Verification items for the finished model (mm, model axes). Face numbers are marked on the shaded views. A direction names the side the tool comes from. Round coordinates to 2 decimals unless told otherwise and drop trailing zeros. Order: outer loops, then holes, each group sorted by start corner. A loop starts at its lowest first (then second) coordinate and runs counter-clockwise, first axis right, second up. Notation, with made-up numbers: M 18,20 L 34,20 A17 cw 34,25 Z; hole C 23,39.25 d6. An arc over 180 degrees is marked long. Return JSON: item names as keys, results as strings. Group by question number.
from build123d import *

# Parameters (mm, degrees)
SKETCH1_R           = 2.5
BOSS_EXTRUDE1_DEPTH = 10


with BuildPart() as part:
    # Sketch1 → Boss-Extrude1 (new body)
    with BuildSketch(Plane.XY):
        with BuildLine():
            Line((-28.989483497, 5.472036177), (-25.856829214, 2.724772104))
            ThreePointArc((-25.856829214, 2.724772104), (-25.874802893, 2.548445649), (-25.891574158, 2.372000766))
            Line((-25.891574158, 2.372000766), (-29.5, 0.288675135))
            Line((-29.5, 0.288675135), (-29.5, -0.288675135))
            Line((-29.5, -0.288675135), (-25.891574158, -2.372000766))
            ThreePointArc((-25.891574158, -2.372000766), (-25.874802893, -2.548445649), (-25.856829214, -2.724772104))
            Line((-25.856829214, -2.724772104), (-28.989483497, -5.472036177))
            Line((-28.989483497, -5.472036177), (-28.876848047, -6.038292822))
            Line((-28.876848047, -6.038292822), (-24.931320427, -7.377618976))
            ThreePointArc((-24.931320427, -7.377618976), (-24.880448729, -7.547401609), (-24.828420824, -7.716833509))
            Line((-24.828420824, -7.716833509), (-27.3649174, -11.022460206))
            Line((-27.3649174, -11.022460206), (-27.143975018, -11.555862303))
            Line((-27.143975018, -11.555862303), (-23.012970034, -12.099719427))
            ThreePointArc((-23.012970034, -12.099719427), (-22.929952873, -12.256315157), (-22.845870145, -12.412341331))
            Line((-22.845870145, -12.412341331), (-24.688732875, -16.149297272))
            Line((-24.688732875, -16.149297272), (-24.367974251, -16.629346476))
            Line((-24.367974251, -16.629346476), (-20.210244109, -16.356834445))
            ThreePointArc((-20.210244109, -16.356834445), (-20.098271787, -16.494225388), (-19.985365489, -16.630849836))
            Line((-19.985365489, -16.630849836), (-21.06377419, -20.6555259))
            Line((-21.06377419, -20.6555259), (-20.6555259, -21.06377419))
            Line((-20.6555259, -21.06377419), (-16.630849836, -19.985365489))
            ThreePointArc((-16.630849836, -19.985365489), (-16.494225388, -20.098271787), (-16.356834445, -20.210244109))
            Line((-16.356834445, -20.210244109), (-16.629346476, -24.367974251))
            Line((-16.629346476, -24.367974251), (-16.149297272, -24.688732875))
            Line((-16.149297272, -24.688732875), (-12.412341331, -22.845870145))
            ThreePointArc((-12.412341331, -22.845870145), (-12.256315157, -22.929952873), (-12.099719427, -23.012970034))
            Line((-12.099719427, -23.012970034), (-11.555862303, -27.143975018))
            Line((-11.555862303, -27.143975018), (-11.022460206, -27.3649174))
            Line((-11.022460206, -27.3649174), (-7.716833509, -24.828420824))
            ThreePointArc((-7.716833509, -24.828420824), (-7.547401609, -24.880448729), (-7.377618976, -24.931320427))
            Line((-7.377618976, -24.931320427), (-6.038292822, -28.876848047))
            Line((-6.038292822, -28.876848047), (-5.472036177, -28.989483497))
            Line((-5.472036177, -28.989483497), (-2.724772104, -25.856829214))
            ThreePointArc((-2.724772104, -25.856829214), (-2.548445649, -25.874802893), (-2.372000766, -25.891574158))
            Line((-2.372000766, -25.891574158), (-0.288675135, -29.5))
            Line((-0.288675135, -29.5), (0.288675135, -29.5))
            Line((0.288675135, -29.5), (2.372000766, -25.891574158))
            ThreePointArc((2.372000766, -25.891574158), (2.548445649, -25.874802893), (2.724772104, -25.856829214))
            Line((2.724772104, -25.856829214), (5.472036177, -28.989483497))
            Line((5.472036177, -28.989483497), (6.038292822, -28.876848047))
            Line((6.038292822, -28.876848047), (7.377618976, -24.931320427))
            ThreePointArc((7.377618976, -24.931320427), (7.547401609, -24.880448729), (7.716833509, -24.828420824))
            Line((7.716833509, -24.828420824), (11.022460206, -27.3649174))
            Line((11.022460206, -27.3649174), (11.555862303, -27.143975018))
            Line((11.555862303, -27.143975018), (12.099719427, -23.012970034))
            ThreePointArc((12.099719427, -23.012970034), (12.256315157, -22.929952873), (12.412341331, -22.845870145))
            Line((12.412341331, -22.845870145), (16.149297272, -24.688732875))
            Line((16.149297272, -24.688732875), (16.629346476, -24.367974251))
            Line((16.629346476, -24.367974251), (16.356834445, -20.210244109))
            ThreePointArc((16.356834445, -20.210244109), (16.494225388, -20.098271787), (16.630849836, -19.985365489))
            Line((16.630849836, -19.985365489), (20.6555259, -21.06377419))
            Line((20.6555259, -21.06377419), (21.06377419, -20.6555259))
            Line((21.06377419, -20.6555259), (19.985365489, -16.630849836))
            ThreePointArc((19.985365489, -16.630849836), (20.098271787, -16.494225388), (20.210244109, -16.356834445))
            Line((20.210244109, -16.356834445), (24.367974251, -16.629346476))
            Line((24.367974251, -16.629346476), (24.688732875, -16.149297272))
            Line((24.688732875, -16.149297272), (22.845870145, -12.412341331))
            ThreePointArc((22.845870145, -12.412341331), (22.929952873, -12.256315157), (23.012970034, -12.099719427))
            Line((23.012970034, -12.099719427), (27.143975018, -11.555862303))
            Line((27.143975018, -11.555862303), (27.3649174, -11.022460206))
            Line((27.3649174, -11.022460206), (24.828420824, -7.716833509))
            ThreePointArc((24.828420824, -7.716833509), (24.880448729, -7.547401609), (24.931320427, -7.377618976))
            Line((24.931320427, -7.377618976), (28.876848047, -6.038292822))
            Line((28.876848047, -6.038292822), (28.989483497, -5.472036177))
            Line((28.989483497, -5.472036177), (25.856829214, -2.724772104))
            ThreePointArc((25.856829214, -2.724772104), (25.874802893, -2.548445649), (25.891574158, -2.372000766))
            Line((25.891574158, -2.372000766), (29.5, -0.288675135))
            Line((29.5, -0.288675135), (29.5, 0.288675135))
            Line((29.5, 0.288675135), (25.891574158, 2.372000766))
            ThreePointArc((25.891574158, 2.372000766), (25.874802893, 2.548445649), (25.856829214, 2.724772104))
            Line((25.856829214, 2.724772104), (28.989483497, 5.472036177))
            Line((28.989483497, 5.472036177), (28.876848047, 6.038292822))
            Line((28.876848047, 6.038292822), (24.931320427, 7.377618976))
            ThreePointArc((24.931320427, 7.377618976), (24.880448729, 7.547401609), (24.828420824, 7.716833509))
            Line((24.828420824, 7.716833509), (27.3649174, 11.022460206))
            Line((27.3649174, 11.022460206), (27.143975018, 11.555862303))
            Line((27.143975018, 11.555862303), (23.012970034, 12.099719427))
            ThreePointArc((23.012970034, 12.099719427), (22.929952873, 12.256315157), (22.845870145, 12.412341331))
            Line((22.845870145, 12.412341331), (24.688732875, 16.149297272))
            Line((24.688732875, 16.149297272), (24.367974251, 16.629346476))
            Line((24.367974251, 16.629346476), (20.210244109, 16.356834445))
            ThreePointArc((20.210244109, 16.356834445), (20.098271787, 16.494225388), (19.985365489, 16.630849836))
            Line((19.985365489, 16.630849836), (21.06377419, 20.6555259))
            Line((21.06377419, 20.6555259), (20.6555259, 21.06377419))
            Line((20.6555259, 21.06377419), (16.630849836, 19.985365489))
            ThreePointArc((16.630849836, 19.985365489), (16.494225388, 20.098271787), (16.356834445, 20.210244109))
            Line((16.356834445, 20.210244109), (16.629346476, 24.367974251))
            Line((16.629346476, 24.367974251), (16.149297272, 24.688732875))
            Line((16.149297272, 24.688732875), (12.412341331, 22.845870145))
            ThreePointArc((12.412341331, 22.845870145), (12.256315157, 22.929952873), (12.099719427, 23.012970034))
            Line((12.099719427, 23.012970034), (11.555862303, 27.143975018))
            Line((11.555862303, 27.143975018), (11.022460206, 27.3649174))
            Line((11.022460206, 27.3649174), (7.716833509, 24.828420824))
            ThreePointArc((7.716833509, 24.828420824), (7.547401609, 24.880448729), (7.377618976, 24.931320427))
            Line((7.377618976, 24.931320427), (6.038292822, 28.876848047))
            Line((6.038292822, 28.876848047), (5.472036177, 28.989483497))
            Line((5.472036177, 28.989483497), (2.724772104, 25.856829214))
            ThreePointArc((2.724772104, 25.856829214), (2.548445649, 25.874802893), (2.372000766, 25.891574158))
            Line((2.372000766, 25.891574158), (0.288675135, 29.5))
            Line((0.288675135, 29.5), (-0.288675135, 29.5))
            Line((-0.288675135, 29.5), (-2.372000766, 25.891574158))
            ThreePointArc((-2.372000766, 25.891574158), (-2.548445649, 25.874802893), (-2.724772104, 25.856829214))
            Line((-2.724772104, 25.856829214), (-5.472036177, 28.989483497))
            Line((-5.472036177, 28.989483497), (-6.038292822, 28.876848047))
            Line((-6.038292822, 28.876848047), (-7.377618976, 24.931320427))
            ThreePointArc((-7.377618976, 24.931320427), (-7.547401609, 24.880448729), (-7.716833509, 24.828420824))
            Line((-7.716833509, 24.828420824), (-11.022460206, 27.3649174))
            Line((-11.022460206, 27.3649174), (-11.555862303, 27.143975018))
            Line((-11.555862303, 27.143975018), (-12.099719427, 23.012970034))
            ThreePointArc((-12.099719427, 23.012970034), (-12.256315157, 22.929952873), (-12.412341331, 22.845870145))
            Line((-12.412341331, 22.845870145), (-16.149297272, 24.688732875))
            Line((-16.149297272, 24.688732875), (-16.629346476, 24.367974251))
            Line((-16.629346476, 24.367974251), (-16.356834445, 20.210244109))
            ThreePointArc((-16.356834445, 20.210244109), (-16.494225388, 20.098271787), (-16.630849836, 19.985365489))
            Line((-16.630849836, 19.985365489), (-20.6555259, 21.06377419))
            Line((-20.6555259, 21.06377419), (-21.06377419, 20.6555259))
            Line((-21.06377419, 20.6555259), (-19.985365489, 16.630849836))
            ThreePointArc((-19.985365489, 16.630849836), (-20.098271787, 16.494225388), (-20.210244109, 16.356834445))
            Line((-20.210244109, 16.356834445), (-24.367974251, 16.629346476))
            Line((-24.367974251, 16.629346476), (-24.688732875, 16.149297272))
            Line((-24.688732875, 16.149297272), (-22.845870145, 12.412341331))
            ThreePointArc((-22.845870145, 12.412341331), (-22.929952873, 12.256315157), (-23.012970034, 12.099719427))
            Line((-23.012970034, 12.099719427), (-27.143975018, 11.555862303))
            Line((-27.143975018, 11.555862303), (-27.3649174, 11.022460206))
            Line((-27.3649174, 11.022460206), (-24.828420824, 7.716833509))
            ThreePointArc((-24.828420824, 7.716833509), (-24.880448729, 7.547401609), (-24.931320427, 7.377618976))
            Line((-24.931320427, 7.377618976), (-28.876848047, 6.038292822))
            Line((-28.876848047, 6.038292822), (-28.989483497, 5.472036177))
        make_face()
        Circle(SKETCH1_R, mode=Mode.SUBTRACT)
    extrude(amount=BOSS_EXTRUDE1_DEPTH)


solid = part.part
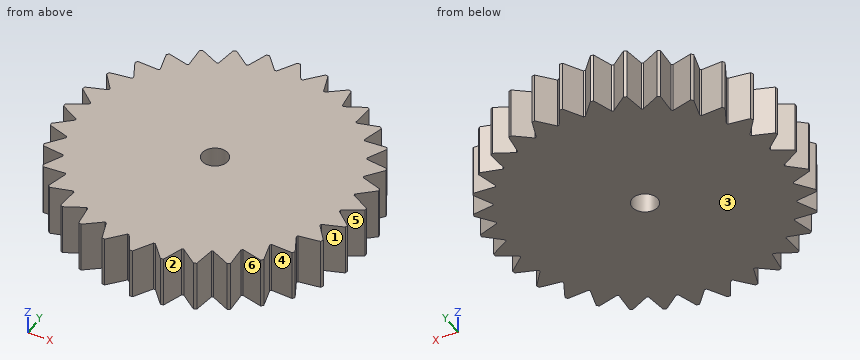
1. Go/stop test with flat-tipped pins: pin 1 (3 mm diameter, centred on x = -17.5, z = 3.5, fed in from -Y); pin 2 (4.5 mm diameter, centred on x = 0, y = 0, fed in from -Z); pin 3 (1.5 mm diameter, centred on y = 20.5, z = 3.5, fed in from -X); pin 4 (1.5 mm diameter, centred on y = -3.5, z = 2.5, fed in from -X). Record where each tip stops, or that it passes through.
2. Draft check along Y on the marked faces 1, 2 and 3. Enter one of: +Y half, -Y half, draft (parallel to the pull), parting line (faces both ways), or undercut.
3. Cross-section at B-B (x = -9). Enter the section's corners in (y, z), plus the area to 3 significant figures.
4. Cross-section at A-A (y = -17.5). Enter the section's corners in (x, z), plus the area to 3 significant figures.
5. Access from +Z, -Z, +X, -X, +Y, -Y to the whole of each face (thin tool, end or side, straight path). Record for the marked faces 4, 5 and 6.
6. Thickness scan on line 1 along Y through (x, z) = (0, 5.75); line 2 along X through (y, z) = (-24, 7.5); line 3 along X through (y, z) = (25, 4.25). Record the ranges inside material, lowest first. Write a range as from..to.
Computed:
{
 "1": {"pin 1": "stops at y = -24.69", "pin 2": "passes through", "pin 3": "stops at x = -21.06", "pin 4": "stops at x = -27.6"},
 "2": {"face 1": "undercut", "face 2": "-Y half", "face 3": "draft"},
 "3": {"outline": "M -25.81,0 L 25.81,0 L 25.81,10 L -25.81,10 Z", "area": "516 mm²"},
 "4": {"outline": "M -20.22,0 L 20.22,0 L 20.22,10 L -20.22,10 Z", "area": "404 mm²"},
 "5": {"face 4": "+Z, -Z", "face 5": "+Z, -Z, +X", "face 6": "+Z, -Z, -Y"},
 "6": {"line 1": "y = -29.5..-2.5, 2.5..29.5", "line 2": "x = -16.61..-14.75, -11.97..11.97, 14.75..16.61", "line 3": "x = -11.84..-7.94, -7.35..7.35, 7.94..11.84"}
}
